from build123d import *

# Parameters (mm, degrees)
F1_DEPTH = 152.4
F1_TAPER = -3


with BuildPart() as f1:
    # F0 (on Front) → F1 (new body)
    with BuildSketch(Plane.XZ):
        with BuildLine():
            Line((384.4163761884, 29.7510090653), (-377.5836238116, 29.7510090653))
            ThreePointArc((-377.5836238116, 29.7510090653), (-431.465160538, 7.4325457917), (-453.7836238116, -46.4489909347))
            Line((-453.7836238116, -46.4489909347), (-453.7836238116, -224.2489909347))
            ThreePointArc((-453.7836238116, -224.2489909347), (-394.2677217487, -367.9330888718), (-250.5836238116, -427.4489909347))
            Line((-250.5836238116, -427.4489909347), (257.4163761884, -427.4489909347))
            ThreePointArc((257.4163761884, -427.4489909347), (401.1004741255, -367.9330888718), (460.6163761884, -224.2489909347))
            Line((460.6163761884, -224.2489909347), (460.6163761884, -46.4489909347))
            ThreePointArc((460.6163761884, -46.4489909347), (438.2979129148, 7.4325457917), (384.4163761884, 29.7510090653))
        make_face()
    extrude(amount=F1_DEPTH, taper=F1_TAPER)


solid = f1.part
Source: CAD feature listing. Evaluate the final solid. Frame: model axes, mm. Coordinates: 2 decimals unless noted, no trailing zeros. Order: outer loops, then holes, each group sorted by start corner. A loop starts at its lowest first (then second) coordinate and runs counter-clockwise, first axis right, second up. Notation, with made-up numbers: M 52.5,2.25 L 89.5,2.25 A17 ccw 89.5,16.25 Z; hole C 17.25,78 d2. An arc over 180 degrees is marked long. Write each question's results on one line, items separated by ' | '. Start each with the question number.
1. Material intervals for L1, parallel to Z at x = 357, y = -122.5; L2, parallel to Z at x = 215, y = -45.5; L3, parallel to X at y = -62, z = -36, sorted ascending.
2. Pin query (flat end, axial travel): pin 1 (2 mm diameter, centred on x = 38.5, y = -29, fed in from -Z); pin 2 (10 mm diameter, centred on x = -8, y = -71.5, fed in from -Z); pin 3 (6 mm diameter, centred on x = -335.5, y = -37.5, fed in from +Z). Return the tip coordinate at first contact, or that it passes through.
3. Section A-A, the plane y = -18. Return the cut outline in (x, z), then the cut area to 3 significant figures.
4. Section C-C, the plane y = -111. Return the cut outline in (x, z), then the cut area to 3 significant figures.
5. Section B-B, the plane x = -30.5. Return the cut outline in (y, z), then the cut area to 3 significant figures.
Solution:
1) L1: -408.7 to 36.17 | L2: -429.83 to 32.14 | L3: -456.34 to 463.18
2) pin 1: z = -429.02 | pin 2: z = -431.46 | pin 3: z = 31.87
3) outline: M -454.73,-224.25 A204.14 ccw -250.58,-428.39 L 257.42,-428.39 A204.14 ccw 461.56,-224.25 L 461.56,-46.45 A77.14 ccw 384.42,30.69 L -377.58,30.69 A77.14 ccw -454.73,-46.45 Z | area: 400,000 mm²
4) outline: M -459.6,-224.25 A209.02 ccw -250.58,-433.27 L 257.42,-433.27 A209.02 ccw 466.43,-224.25 L 466.43,-46.45 A82.02 ccw 384.42,35.57 L -377.58,35.57 A82.02 ccw -459.6,-46.45 Z | area: 413,000 mm²
5) outline: M -152.4,-435.44 L 0,-427.45 L 0,29.75 L -152.4,37.74 Z | area: 70,900 mm²
